from build123d import *

# Parameters (mm, degrees)
SKETCH1_W                      = 104
SKETCH1_H                      = 50
BOSS_EXTRUDE1_DEPTH            = 10
SKETCH2_W                      = 104
SKETCH2_H                      = 50
BOSS_EXTRUDE2_DEPTH            = 25
SKETCH3_W                      = 14.6
SKETCH3_H                      = 50
BOSS_EXTRUDE3_DEPTH            = 25
CUT_EXTRUDE1_DEPTH             = 113.543324991
CUT_EXTRUDE1_DEPTH_BACK        = 113.543324991
SKETCH4_R                      = 1.7
CUT_EXTRUDE2_DEPTH             = 68.483331275
CUT_EXTRUDE2_DEPTH_BACK        = 68.483331275
SKETCH5_R                      = 2
CUT_EXTRUDE4_REACH             = 82.181
SKETCH8_R                      = 3.5
CUT_EXTRUDE4_DIRECTION_2_DEPTH = 81.181045142
FILLET1_R                      = 2.5
CUT_EXTRUDE6_REACH             = 82.181
CUT_EXTRUDE6_DIRECTION_2_DEPTH = 81.181045142
CUT_EXTRUDE7_REACH             = 82.181
SKETCH10_W                     = 25
SKETCH10_H                     = 10
CUT_EXTRUDE7_DIRECTION_2_DEPTH = 81.181045142


with BuildPart() as part:
    # Sketch1 → Boss-Extrude1 (new body)
    with BuildSketch(Plane(origin=(0, 0, 0), x_dir=(1, 0, 0), z_dir=(0, 1, 0))):
        Rectangle(SKETCH1_W, SKETCH1_H)
    extrude(amount=BOSS_EXTRUDE1_DEPTH)

    # Sketch2 → Boss-Extrude2 (add)
    with BuildSketch(Plane.XZ):
        Rectangle(SKETCH2_W, SKETCH2_H)
        Polygon((-45.5, 13.5), (-45.5, 0), (-45.5, -13.5), (0, -13.5), (45.5, -13.5), (45.5, 0), (45.5, 13.5), (0, 13.5), align=None, mode=Mode.SUBTRACT)
    extrude(amount=BOSS_EXTRUDE2_DEPTH)

    # Sketch3 → Boss-Extrude3 (add)
    with BuildSketch(Plane(origin=(0, 10, 0), x_dir=(1, 0, 0), z_dir=(0, 1, 0))):
        with Locations((-44.7, 0)):
            Rectangle(SKETCH3_W, SKETCH3_H)
        with Locations((44.7, 0)):
            Rectangle(SKETCH3_W, SKETCH3_H)
    extrude(amount=BOSS_EXTRUDE3_DEPTH)

    # Sketch4 → Cut-Extrude1 (cut, two sides: drawn at the far end of the back side and taken through both)
    with BuildSketch(Plane(origin=(52, 0, 0), x_dir=(0, 0, -1), z_dir=(1, 0, 0)).offset(-CUT_EXTRUDE1_DEPTH_BACK)):
        with Locations((17, 27)):
            Circle(SKETCH4_R)
        with Locations((-17, 27)):
            Circle(SKETCH4_R)
    extrude(amount=CUT_EXTRUDE1_DEPTH + CUT_EXTRUDE1_DEPTH_BACK, mode=Mode.SUBTRACT)

    # Sketch5 → Cut-Extrude2 (cut, two sides: drawn at the far end of the back side and taken through both)
    with BuildSketch(Plane(origin=(0, 10, 0), x_dir=(1, 0, 0), z_dir=(0, 1, 0)).offset(-CUT_EXTRUDE2_DEPTH_BACK)):
        with Locations(Location((-22.5, 0, 0), (0, 0, 270))):
            Circle(SKETCH5_R)
        with Locations(Location((22.5, 0, 0), (0, 0, 270))):
            Circle(SKETCH5_R)
    extrude(amount=CUT_EXTRUDE2_DEPTH + CUT_EXTRUDE2_DEPTH_BACK, mode=Mode.SUBTRACT)

    # Sketch8 → Cut-Extrude4 (cut, up to next)
    with BuildSketch(Plane.XY.offset(25), mode=Mode.PRIVATE) as cut_extrude4_sk1:
        with Locations(Location((0, -10.65, 0), (0, 0, 180))):
            Circle(SKETCH8_R)
    cut_extrude4_tool1 = extrude(cut_extrude4_sk1.sketch, amount=-CUT_EXTRUDE4_REACH, mode=Mode.PRIVATE) & part.part
    add(cut_extrude4_tool1.solids().sort_by_distance((0, -10.65, 25))[0], mode=Mode.SUBTRACT)

    # Sketch8 → Cut-Extrude4 direction 2 (cut)
    with BuildSketch(Plane.XY.offset(25)):
        with Locations(Location((0, -10.65, 0), (0, 0, 180))):
            Circle(SKETCH8_R)
    extrude(amount=CUT_EXTRUDE4_DIRECTION_2_DEPTH, mode=Mode.SUBTRACT)

    # Fillet1
    fillet1_edges = [part.edges().sort_by_distance(p)[0] for p in [
        (-52, 35, 0),
        (-37.4, 35, 0),
        (37.4, 35, 0),
        (52, 35, 0),
        (-52, 5, 25),
        (-52, 5, -25),
        (52, 5, -25),
        (52, 5, 25),
    ]]
    fillet(fillet1_edges, radius=FILLET1_R)

    # Sketch9 → Cut-Extrude6 (cut, up to next)
    with BuildSketch(Plane(origin=(0, 0, -25), x_dir=(-1, 0, 0), z_dir=(0, 0, -1)), mode=Mode.PRIVATE) as cut_extrude6_sk1:
        Polygon((-33, -6), (-33, -16), (0, -16), (33, -16), (33, -6), (0, -6), align=None)
    cut_extrude6_tool1 = extrude(cut_extrude6_sk1.sketch, amount=-CUT_EXTRUDE6_REACH, mode=Mode.PRIVATE) & part.part
    add(cut_extrude6_tool1.solids().sort_by_distance((0, -11, -25))[0], mode=Mode.SUBTRACT)

    # Sketch9 → Cut-Extrude6 direction 2 (cut)
    with BuildSketch(Plane(origin=(0, 0, -25), x_dir=(-1, 0, 0), z_dir=(0, 0, -1))):
        Polygon((-33, -6), (-33, -16), (0, -16), (33, -16), (33, -6), (0, -6), align=None)
    extrude(amount=CUT_EXTRUDE6_DIRECTION_2_DEPTH, mode=Mode.SUBTRACT)

    # Sketch10 → Cut-Extrude7 (cut, up to next)
    with BuildSketch(Plane.XY.offset(25), mode=Mode.PRIVATE) as cut_extrude7_sk1:
        with Locations((-20.5, -11)):
            Rectangle(SKETCH10_W, SKETCH10_H)
    cut_extrude7_tool1 = extrude(cut_extrude7_sk1.sketch, amount=-CUT_EXTRUDE7_REACH, mode=Mode.PRIVATE) & part.part
    # Sketch10 → Cut-Extrude7 (cut, up to next)
    with BuildSketch(Plane.XY.offset(25), mode=Mode.PRIVATE) as cut_extrude7_sk2:
        with Locations((20.5, -11)):
            Rectangle(SKETCH10_W, SKETCH10_H)
    cut_extrude7_tool2 = extrude(cut_extrude7_sk2.sketch, amount=-CUT_EXTRUDE7_REACH, mode=Mode.PRIVATE) & part.part
    add(cut_extrude7_tool1.solids().sort_by_distance((-20.5, -11, 25))[0], mode=Mode.SUBTRACT)
    add(cut_extrude7_tool2.solids().sort_by_distance((20.5, -11, 25))[0], mode=Mode.SUBTRACT)

    # Sketch10 → Cut-Extrude7 direction 2 (cut)
    with BuildSketch(Plane.XY.offset(25)):
        with Locations((-20.5, -11)):
            Rectangle(SKETCH10_W, SKETCH10_H)
        with Locations((20.5, -11)):
            Rectangle(SKETCH10_W, SKETCH10_H)
    extrude(amount=CUT_EXTRUDE7_DIRECTION_2_DEPTH, mode=Mode.SUBTRACT)


solid = part.part
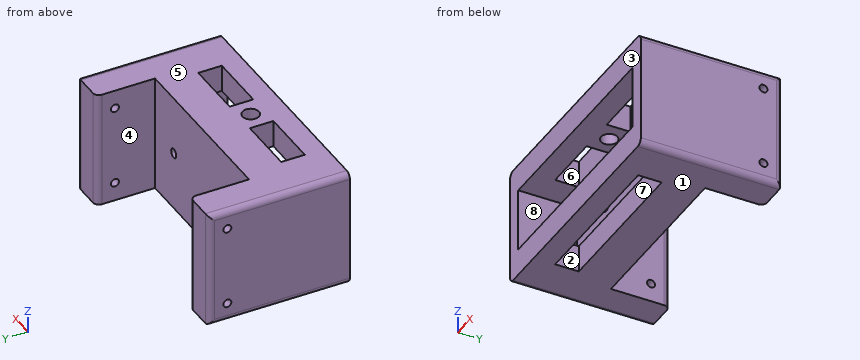
Part model, mm, in its own coordinate system. Face numbers are marked on the shaded views. A direction names the side the tool comes from. Coordinates: 2 decimals unless noted, no trailing zeros. Loops run counter-clockwise (first coordinate to the right, second up) from the corner with the lowest first, then second, coordinate; pieces in that order, holes last. Notation, with made-up numbers: (14, -31.75) -> (67, -31.75) arc R24 cw to (67, -17.75) -> close; hole circle Ø3 at (-30.75, 11.25). An arc over 180 degrees is marked (long way). Use a Markdown table: item, result. Add a question column.
Item 1: Band-saw the part on D-D on y = -10.65. Write the cut outline in (x, z).
Item 2: Pull direction Y, two halves, no side cores. Call the marked faces 1, 2 and 3: +Y half, -Y half, draft (parallel to the pull), parting line (faces both ways), or undercut.
Item 3: Band-saw the part on C-C on x = -22.5. Write the cut outline in (y, z), plus the area to 3 significant figures.
Item 4: Probe probe 1 along Y at (x, z) = (16.5, -21.5); probe 2 along Y at (x, z) = (48, -17); probe 3 along Z at (x, y) = (-22.5, 2.75). List the from-to ranges inside material, lowest first.
Item 5: Flat gauge pins, fed straight in: P1, Ø3.5, axis at x = 24.5, z = 21, coming from the +Y side; P2, Ø3, axis at y = 27, z = 17, coming from the +X side; P3, Ø20, axis at x = 21, y = -8, coming from the +Z side; P4, Ø13.5, axis at x = 22, z = 5.5, coming from the -Y side. Where does each tip first touch, or does it go through?
Item 6: Which spindle directions (+Z, -Z, +X, -X, +Y, -Y) get a long thin tool onto all of the face, cutting with end or side? Do the marked faces 4, 5, 6, 7 and 8. Say none if no direction does.
Item 7: Band-saw the part on B-B on y = 18. Write the cut outline in (x, z), plus the area to 3 significant figures.
Item 8: Band-saw the part on A-A on z = -17. Write the cut outline in (x, y).
Geometry says:
| question | item | result |
|---|---|---|
| 1 | outline | (-52, -22.5) arc R2.5 ccw to (-49.5, -25) -> (-33, -25) -> (-33, -13.5) -> (-45.5, -13.5) -> (-45.5, 13.5) -> (-33, 13.5) -> (-33, 25) -> (-49.5, 25) arc R2.5 ccw to (-52, 22.5) -> close; (-8, 13.5) -> (-3.5, 13.5) -> (-3.5, 25) -> (-8, 25) -> close; (3.5, 13.5) -> (8, 13.5) -> (8, 25) -> (3.5, 25) -> close; (33, -25) -> (49.5, -25) arc R2.5 ccw to (52, -22.5) -> (52, 22.5) arc R2.5 ccw to (49.5, 25) -> (33, 25) -> (33, 13.5) -> (45.5, 13.5) -> (45.5, -13.5) -> (33, -13.5) -> close |
| 2 | face 1 | draft |
| 2 | face 2 | undercut |
| 2 | face 3 | -Y half |
| 3 | outline | (-25, -25) -> (-16, -25) -> (-16, -13.5) -> (-25, -13.5) -> close; (-25, 13.5) -> (-16, 13.5) -> (-16, 25) -> (-25, 25) -> close; (-6, -25) -> (10, -25) -> (10, -2) -> (0, -2) -> (0, -13.5) -> (-6, -13.5) -> close; (-6, 13.5) -> (0, 13.5) -> (0, 2) -> (10, 2) -> (10, 25) -> (-6, 25) -> close |
| 3 | area | 805 mm² |
| 4 | probe 1 | -25 to -16, -6 to 10 |
| 4 | probe 2 | -25 to 25.3, 28.7 to 35 |
| 4 | probe 3 | -25 to -2, 2 to 25 |
| 5 | P1 | y = 10 |
| 5 | P2 | through |
| 5 | P3 | z = 25 |
| 5 | P4 | y = 0 |
| 6 | face 4 | +Z, -Z, +Y |
| 6 | face 5 | +Z, +X, -X, +Y, -Y |
| 6 | face 6 | +Z, -Z |
| 6 | face 7 | -Z |
| 6 | face 8 | -Y |
| 7 | outline | (-52, -22.5) arc R2.5 ccw to (-49.5, -25) -> (-37.4, -25) -> (-37.4, 25) -> (-49.5, 25) arc R2.5 ccw to (-52, 22.5) -> close; (37.4, -25) -> (49.5, -25) arc R2.5 ccw to (52, -22.5) -> (52, 22.5) arc R2.5 ccw to (49.5, 25) -> (37.4, 25) -> close |
| 7 | area | 1,450 mm² |
| 8 | outline | (-52, -25) -> (52, -25) -> (52, 25.3) -> (37.4, 25.3) -> (37.4, 10) -> (-37.4, 10) -> (-37.4, 25.3) -> (-52, 25.3) -> close; (-52, 28.7) -> (-37.4, 28.7) -> (-37.4, 32.5) arc R2.5 ccw to (-39.9, 35) -> (-49.5, 35) arc R2.5 ccw to (-52, 32.5) -> close; (37.4, 28.7) -> (52, 28.7) -> (52, 32.5) arc R2.5 ccw to (49.5, 35) -> (39.9, 35) arc R2.5 ccw to (37.4, 32.5) -> close; hole (-33, -16) -> (33, -16) -> (33, -6) -> (-33, -6) -> close |
